Can you work these out from the drawing? Everything is in mm from the part's minimum corner. Round coordinates to 2 decimals unless told otherwise and drop trailing zeros. Loops run counter-clockwise (first coordinate to the right, second up) from the corner with the lowest first, then second, coordinate; pieces in that order, holes last. Notation, with made-up numbers: (-26, 81) -> (23, 81) arc R7 cw to (23, 89) -> close; hole circle Ø4 at (-25.5, 47.25). An arc over 180 degrees is marked (long way). One line per item, written item: value.
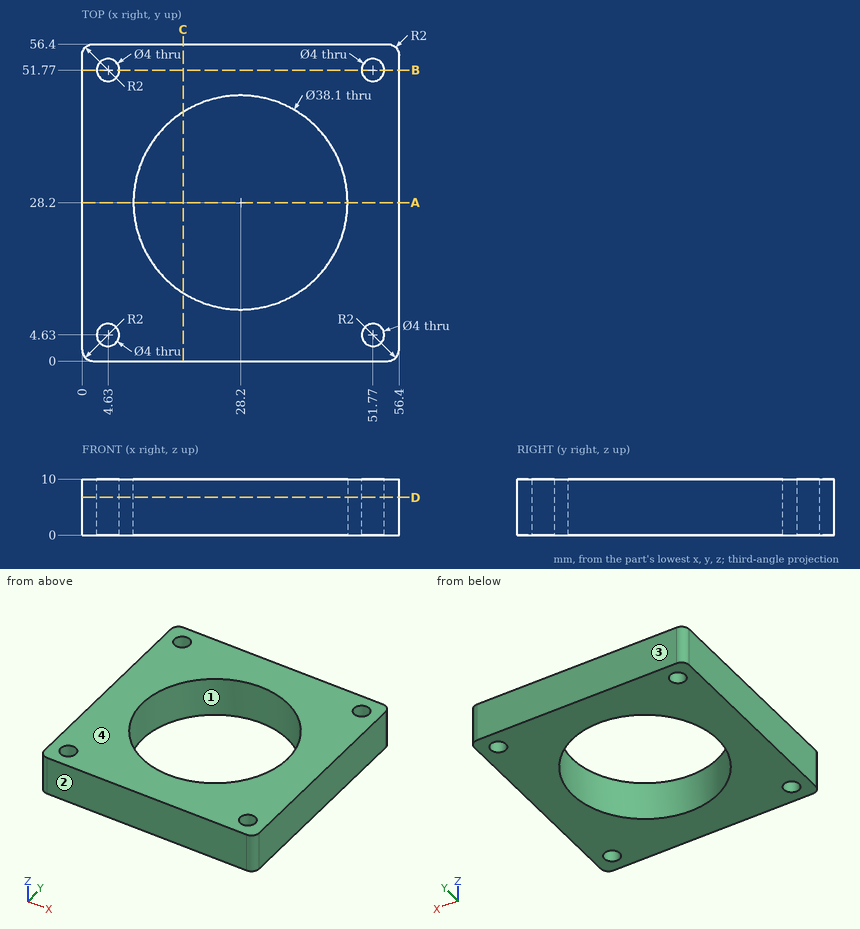
(1) If we section it at A-A, the plane y = 28.2: Please give me the cut outline in (x, z), then the cut area to 3 significant figures.
Recorded:
outline: (0, 0) -> (9.15, 0) -> (9.15, 10) -> (0, 10) -> close; (47.25, 0) -> (56.4, 0) -> (56.4, 10) -> (47.25, 10) -> close
area: 183 mm²
(2) If we section it at D-D, the plane z = 6.75: Please give me the cut outline in (x, y).
Recorded:
outline: (0, 2) arc R2 ccw to (2, 0) -> (54.4, 0) arc R2 ccw to (56.4, 2) -> (56.4, 54.4) arc R2 ccw to (54.4, 56.4) -> (2, 56.4) arc R2 ccw to (0, 54.4) -> close; hole circle Ø4 at (4.63, 4.63); hole circle Ø4 at (4.63, 51.77); hole circle Ø38.1 at (28.2, 28.2); hole circle Ø4 at (51.77, 4.63); hole circle Ø4 at (51.77, 51.77)
(3) If we section it at B-B, the plane y = 51.77: Please give me the cut outline in (x, z).
Recorded:
outline: (0, 0) -> (2.63, 0) -> (2.63, 10) -> (0, 10) -> close; (6.63, 0) -> (49.77, 0) -> (49.77, 10) -> (6.63, 10) -> close; (53.77, 0) -> (56.4, 0) -> (56.4, 10) -> (53.77, 10) -> close
(4) If we section it at C-C, the plane x = 18: Please give me the cut outline in (y, z).
Recorded:
outline: (0, 0) -> (12.11, 0) -> (12.11, 10) -> (0, 10) -> close; (44.29, 0) -> (56.4, 0) -> (56.4, 10) -> (44.29, 10) -> close
(5) Thinking about a two-plate mould opening in Y: for the marked faces 1, 2, 3 and 4, which applies, released by +Y, released by -Y, zero draft, split by the parting line, or undercut?
Recorded:
face 1: undercut
face 2: released by -Y
face 3: released by +Y
face 4: zero draft
(6) If I drill on L1, parallel to Y at x = 4.63, z = 5.25; L2, parallel to X at y = 28, z = 4.25, over which ranges is the centre line in solid material (lowest first)?
Recorded:
L1: 0 to 2.63, 6.63 to 49.77, 53.77 to 56.4
L2: 0 to 9.15, 47.25 to 56.4
